```python
from build123d import *

# Parameters (mm, degrees)
BOSS_EXTRUDE1_DEPTH     = 15
SKETCH2_R               = 2.5
BOSS_EXTRUDE2_DEPTH     = 1
CUT_EXTRUDE1_DEPTH      = 3
CUT_EXTRUDE5_DEPTH      = 2
CUT_EXTRUDE5_DEPTH_BACK = 3
SKETCH5_W               = 1.356176493
SKETCH5_H               = 3
CUT_EXTRUDE6_DEPTH      = 3
CUT_EXTRUDE11_DEPTH     = 20
CUT_EXTRUDE12_DEPTH     = 1


with BuildPart() as part:
    # Sketch1 → Boss-Extrude1 (new body)
    with BuildSketch(Plane(origin=(0, 0, 0), x_dir=(1, 0, 0), z_dir=(0, 1, 0))):
        Polygon((53.231444905, 93.562909441), (55.368661466, 80.762909441), (59.368661466, 80.762909441), (59.368661466, 66.562909441), (55.368661466, 66.562909441), (53.231444905, 53.762909441), (25.231444905, 53.762909441), (25.231444905, 58.012909441), (42.701133317, 58.012909441), (42.701133317, 66.512909441), (41.344956824, 66.512909441), (41.344956824, 70.012909441), (12.018661466, 71.012909441), (12.018661466, 76.312909441), (41.344956824, 77.312909441), (41.344956824, 80.812909441), (42.701133317, 80.812909441), (42.701133317, 89.312909441), (25.231444905, 89.312909441), (25.231444905, 93.562909441), align=None)
    extrude(amount=BOSS_EXTRUDE1_DEPTH)

    # Sketch2 → Boss-Extrude2 (add)
    with BuildSketch(Plane.XZ):
        with Locations((42.701133317, -73.662909441)):
            Circle(SKETCH2_R)
    extrude(amount=BOSS_EXTRUDE2_DEPTH)

    # Sketch3 → Cut-Extrude1 (cut)
    with BuildSketch(Plane(origin=(0, 0, 0), x_dir=(-1, 0, 0), z_dir=(0, -1, 0))):
        with BuildLine():
            Line((-42.701133317, 80.812909441), (-55.368661466, 80.762909441))
            Line((-55.368661466, 80.762909441), (-59.368661466, 80.762909441))
            Line((-59.368661466, 80.762909441), (-59.368661466, 66.562909441))
            Line((-59.368661466, 66.562909441), (-41.344956824, 66.512909441))
            Line((-41.344956824, 66.512909441), (-41.344956824, 70.012909441))
            Line((-41.344956824, 70.012909441), (-41.344956824, 71.562722468))
            ThreePointArc((-41.344956824, 71.562722468), (-45.201133317, 73.662909441), (-41.344956824, 75.763096414))
            Line((-41.344956824, 75.763096414), (-41.344956824, 77.312909441))
            Line((-41.344956824, 77.312909441), (-41.344956824, 80.812909441))
            Line((-41.344956824, 80.812909441), (-42.701133317, 80.812909441))
        make_face()
    extrude(amount=-CUT_EXTRUDE1_DEPTH, mode=Mode.SUBTRACT)

    # Sketch4 → Cut-Extrude5 (cut, two sides)
    with BuildSketch(Plane.XZ) as cut_extrude5_sk:
        with BuildLine():
            Line((12.018661466, -76.312909441), (41.344956824, -77.312909441))
            Line((41.344956824, -77.312909441), (41.344956824, -77.220900459))
            Line((41.344956824, -77.220900459), (41.344956824, -75.763096414))
            ThreePointArc((41.344956824, -75.763096414), (40.201133317, -73.662909441), (41.344956824, -71.562722468))
            Line((41.344956824, -71.562722468), (41.344956824, -70.012909441))
            Line((41.344956824, -70.012909441), (12.018661466, -71.012909441))
            Line((12.018661466, -71.012909441), (12.018661466, -76.312909441))
        make_face()
    extrude(amount=CUT_EXTRUDE5_DEPTH, mode=Mode.SUBTRACT)
    extrude(cut_extrude5_sk.sketch, amount=-CUT_EXTRUDE5_DEPTH_BACK, mode=Mode.SUBTRACT)

    # Sketch5 → Cut-Extrude6 (cut)
    with BuildSketch(Plane.XY.offset(-66.512909441)):
        with Locations((42.023045071, 1.5)):
            Rectangle(SKETCH5_W, SKETCH5_H)
    extrude(amount=-CUT_EXTRUDE6_DEPTH, mode=Mode.SUBTRACT)

    # Sketch7 → Cut-Extrude11 (cut)
    with BuildSketch(Plane.ZY.offset(-42.701133317)):
        Polygon((-66.516671643, 0), (-67.290586566, 0), (-67.290586566, 3), (-66.512909441, 3), (-58.012909441, 0), align=None)
        Polygon((-89.312909441, 0), (-80.812909441, 0), (-79.713237651, 0), (-79.713237651, 3), (-80.812909441, 3), align=None)
    extrude(amount=-CUT_EXTRUDE11_DEPTH, mode=Mode.SUBTRACT)

    # Sketch11 → Cut-Extrude12 (cut)
    with BuildSketch(Plane.XZ.offset(-3)):
        with BuildLine():
            Line((41.344956824, -77.312909441), (41.344956824, -75.763096414))
            ThreePointArc((41.344956824, -75.763096414), (40.201133317, -73.662909441), (41.344956824, -71.562722468))
            Line((41.344956824, -71.562722468), (41.344956824, -70.012909441))
            Line((41.344956824, -70.012909441), (12.018661466, -71.012909441))
            Line((12.018661466, -71.012909441), (12.018661466, -76.312909441))
            Line((12.018661466, -76.312909441), (41.344956824, -77.312909441))
        make_face()
    extrude(amount=-CUT_EXTRUDE12_DEPTH, mode=Mode.SUBTRACT)


solid = part.part
```
The model under review builds one solid part; all positions refer to its coordinate system, in mm. A direction names the side the tool comes from. Round coordinates to 2 decimals unless told otherwise and drop trailing zeros. Loops run counter-clockwise (first coordinate to the right, second up) from the corner with the lowest first, then second, coordinate; pieces in that order, holes last.
1) Consider section B-B on y = 9.75. State the section outline as (x, z) points.
Values follow:
outline: (12.02, -76.31) - (41.34, -77.31) - (41.34, -80.81) - (42.7, -80.81) - (42.7, -89.31) - (25.23, -89.31) - (25.23, -93.56) - (53.23, -93.56) - (55.37, -80.76) - (59.37, -80.76) - (59.37, -66.56) - (55.37, -66.56) - (53.23, -53.76) - (25.23, -53.76) - (25.23, -58.01) - (42.7, -58.01) - (42.7, -66.51) - (41.34, -66.51) - (41.34, -70.01) - (12.02, -71.01) - close
2) Consider section D-D on z = -60.5. State the section outline as (x, y) points.
Values follow:
outline: (42.7, 0.88) - (54.36, 0.88) - (54.36, 15) - (42.7, 15) - close
3) Wall thickness on line 1 along Z through (x, y) = (41.5, 6.5); line 2 along Z through (x, y) = (40.5, 0.25); line 3 along Y through (x, z) = (22.5, -72): over which ranges is each line inside the solid? List them lowest first.
Values follow:
line 1: z = -93.56 to -89.31, -80.81 to -66.51, -58.01 to -53.76
line 2: z = -93.56 to -89.31, -74.85 to -72.48, -58.01 to -53.76
line 3: y = 4 to 15
4) Consider section C-C on z = -69.5. State the section outline as (x, y) points, then the cut area to 3 significant figures.
Values follow:
outline: (41.34, 3) - (59.37, 3) - (59.37, 15) - (41.34, 15) - close
area: 216 mm2
5) The part is to be moulded in two halves that separate along Z. For faces 1 (the face through (40.736, 1.465, -72.117)), 2 (the face through (57, 9, -66.563)), 3 (the face through (54.285, 7.395, -87.253)), say which applies: pulls with the +Z half, pulls with the -Z half, needs draft (parallel to the pull), parting line crosses it, or undercut.
Values follow:
face 1: undercut
face 2: pulls with the +Z half
face 3: pulls with the -Z half
6) Clearance check with flat-ended pins moving along their axes: P1, Ø1.5, axis at x = 48.5, z = -65, coming from the -Y side; P2, Ø1.2, axis at x = 58.5, y = 6.5, coming from the -Z side; P3, Ø4.5, axis at y = 4.5, z = -91, coming from the -X side; P4, Ø1, axis at y = 1, z = -79.5, coming from the +X side (1 decimal). State where each tip first meets the part, or that it passes through.
Values follow:
P1: stops at y = 2.2
P2: stops at z = -80.76
P3: stops at x = 25.23
P4: passes through
7) Tool access review of faces 4 (the face through (57, 9, -80.763)), 5 (the face through (25.231, 7, -56)), 6 (the face through (42, 9, -80.813)): name each direction out of +Z, -Z, +X, -X, +Y, -Y from which nothing blocks a thin tool from reaching the whole face with its end or side.
Values follow:
face 4: -Z, +X, +Y, -Y
face 5: +Z, -X, +Y, -Y
face 6: -X, +Y, -Y
8) Consider section A-A on x = 48. State the section outline as (y, z) points, then the cut area to 3 significant figures.
Values follow:
outline: (0, -93.56) - (15, -93.56) - (15, -53.76) - (0, -53.76) - (0, -58.01) - (3, -66.51) - (3, -80.81) - (0, -89.31) - close
area: 529 mm2
